Check sheet for the drawn part. Datum: minimum x, y, z corner. Units: mm. A direction names the side the tool comes from. Give positions to 0.01 mm unless a question says otherwise; leave off trailing zeros. Loops run counter-clockwise (first coordinate to the right, second up) from the corner with the lowest first, then second, coordinate; pieces in that order, holes last. Notation, with made-up numbers: (56, -37.75) - (99, -37.75) arc R17 ccw to (99, -30.75) - close; hole circle Ø1 at (79.5, 71.5). An arc over 180 degrees is marked (long way). One line per item, written item: value. Start each with the question number.
1. Mould release check, pull along Y, two halves, no side actions. Record for the marked faces 6, 7 and 8: pulls with the +Y half, pulls with the -Y half, needs draft (parallel to the pull), parting line crosses it, or undercut.
2. Sectioned sample at D-D (y = 40.05). Record the cut outline in (x, z) (1 decimal), plus the area to 3 significant figures.
3. Sectioned sample at A-A (y = 25.05). Record the cut outline in (x, z), plus the area to 3 significant figures.
4. Access from +Z, -Z, +X, -X, +Y, -Y to the whole of each face (thin tool, end or side, straight path). Record for the marked faces 1, 2, 3, 4 and 5.
5. Gauge pin test, flat ends, axial feed: pin 1 (3 mm diameter, centred on x = 48, z = 5.5, fed in from -Y); pin 2 (1.1 mm diameter, centred on y = 2.5, z = 4.5, fed in from +X); pin 3 (3 mm diameter, centred on x = 49, z = 4.5, fed in from +Y); pin 4 (10 mm diameter, centred on x = 22, y = 32, fed in from -Z). Record the tip position at first contact, or that the pin passes through.
6. Scan lines: L1, parallel to Y at x = 10, z = 14 (1 decimal); L2, parallel to Y at x = 25.05, z = 7; L3, parallel to X at y = 24.5, z = 9.25. Record each from-to range of solid material in increasing order. Write a range as [from, to].
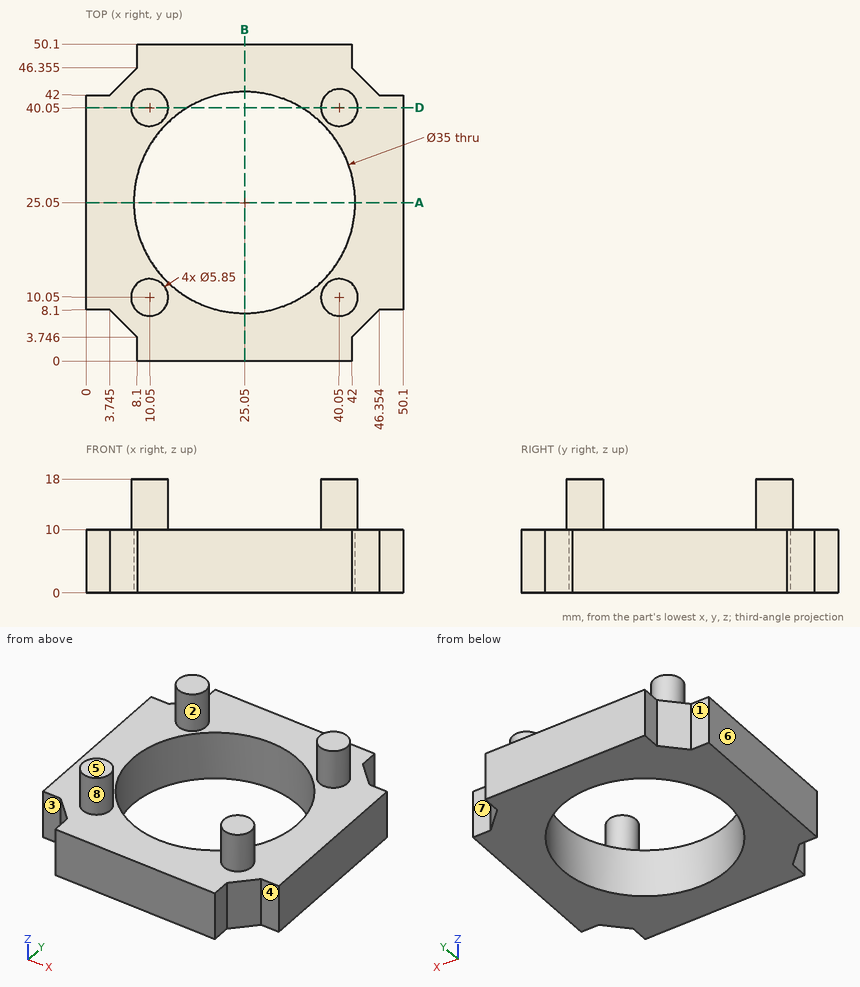
Results are:
1. face 6: needs draft
1. face 7: pulls with the +Y half
1. face 8: undercut
2. outline: (0, 0) - (16, 0) - (16, 10) - (13, 10) - (13, 18) - (7.1, 18) - (7.1, 10) - (0, 10) - close; (34.1, 0) - (50.1, 0) - (50.1, 10) - (43, 10) - (43, 18) - (37.1, 18) - (37.1, 10) - (34.1, 10) - close
2. area: 414 mm^2
3. outline: (0, 0) - (7.55, 0) - (7.55, 10) - (0, 10) - close; (42.55, 0) - (50.1, 0) - (50.1, 10) - (42.55, 10) - close
3. area: 151 mm^2
4. face 1: +Z, -Z, -X, +Y
4. face 2: +Z
4. face 3: +Z, -Z, -X, -Y
4. face 4: +Z, -Z, +X, -Y
4. face 5: +Z, +X, -X, +Y, -Y
5. pin 1: stops at y = 8.1
5. pin 2: stops at x = 42
5. pin 3: stops at y = 42
5. pin 4: passes through
6. L1: y = [7.1, 13], [37.1, 43]
6. L2: y = [0, 7.55], [42.55, 50.1]
6. L3: x = [0, 7.56], [42.54, 50.1]
